Check sheet for the modelled part. Datum: model origin and axes. Units: mm. A direction names the side the tool comes from. Give positions to 0.01 mm unless a question says otherwise; leave off trailing zeros. Loops run counter-clockwise (first coordinate to the right, second up) from the corner with the lowest first, then second, coordinate; pieces in that order, holes last. Notation, with made-up numbers: (57.5, 81.5) - (110.5, 81.5) arc R30 ccw to (110.5, 110.5) - close; hole circle Ø3 at (-25.5, -28). An arc over 180 degrees is marked (long way). Use CSV: the item, a comma, the result in double quotes.
Autodesk Inventor part; units mm, degrees
ref_plane "ANBAU_XY" through (0, 0, -15.2) normal (0, -1, 0) x (1, 0, 0)
ref_plane "ANBAU_YZ" through (0, 0, -15.2) normal (1, 0, 0) x (0, 0, 1)
ref_plane "ANBAU_ZX" through (0, 0, -15.2) normal (0, 0, 1) x (0, -1, 0)
sketch "Sketch_1" plane through (0, 0, 0) normal (1, 0, 0) x (0, 1, 0)
  line L0 (22, 5.4) -> (-20.8, 5.4)
  arc A0 (-20.8, 5.4) -> (-21, 5.2) centre (-20.8, 5.2) ccw
  line L1 (-21, 5.2) -> (-21, 1.1788)
  arc A1 (-21, 1.1788) -> (-20.9463, 1.0424) centre (-20.8, 1.1788) ccw
  line L2 (-20.9463, 1.0424) -> (-20.419, 0.477)
  arc A2 (-20.419, 0.477) -> (-19.322, 0) centre (-19.322, 1.5) ccw
  line L3 (-19.322, 0) -> (21.2, 0)
  line L4 (21.2, 0) -> (21.2, -3.3)
  line L5 (21.2, -3.3) -> (21.6171, -3.3)
  line L6 (21.6171, -3.3) -> (22.1063, -2.2509)
  arc A3 (22.1063, -2.2509) -> (22.2, -1.8283) centre (21.2, -1.8283) ccw
  line L7 (22.2, -1.8283) -> (22.2, 5.2)
  arc A4 (22.2, 5.2) -> (22, 5.4) centre (22, 5.2) ccw
extrude "Extrusion1" add sketch "Sketch_1" along normal mid plane 8
sketch "Sketch_2" plane through (0, 0, 0) normal (1, 0, 0) x (0, 1, 0)
  line L0 (15, 4.2) -> (15, 5.4)
  line L1 (15, 5.4) -> (18.05, 5.4)
  line L2 (18.05, 5.4) -> (18.05, 4.2)
  line L3 (18.05, 4.2) -> (15, 4.2)
  line L4 (15, 4.2) -> (15, 5.4)
revolve "Revolution1" cut sketch "Sketch_2" angle 360 about axis through (0, 15, 4.2) along (0, 0, -1)
sketch "Sketch_3" plane through (0, 0, 0) normal (1, 0, 0) x (0, 1, 0)
  line L0 (-15, 4.2) -> (-15, 5.4)
  line L1 (-15, 5.4) -> (-11.95, 5.4)
  line L2 (-11.95, 5.4) -> (-11.95, 4.2)
  line L3 (-11.95, 4.2) -> (-15, 4.2)
  line L4 (-15, 4.2) -> (-15, 5.4)
revolve "Revolution2" cut sketch "Sketch_3" angle 360 about axis through (0, -15, 4.2) along (0, 0, -1)
sketch "Sketch_6" plane through (0, -21.6, 0) normal (0, 1, 0) x (1, 0, 0)
  arc A0 (-1.7301, -0.5774) -> (-2.6364, 0) centre (-2.6364, -1) ccw
  line L0 (-1.7301, -0.5774) -> (-1.2427, -1.6226)
  arc A1 (-1.2427, -1.6226) -> (-0.3364, -2.2) centre (-0.3364, -1.2) ccw
  line L1 (-0.3364, -2.2) -> (0.3364, -2.2)
  arc A2 (0.3364, -2.2) -> (1.2427, -1.6226) centre (0.3364, -1.2) ccw
  line L2 (1.2427, -1.6226) -> (1.7301, -0.5774)
  arc A3 (2.6364, 0) -> (1.7301, -0.5774) centre (2.6364, -1) ccw
  line L3 (2.6364, 0) -> (-2.6364, 0)
extrude "Extrusion2" cut sketch "Sketch_6" along normal blind 42.8
sketch "Sketch_4" plane through (0, 0, 0) normal (1, 0, 0) x (0, 1, 0)
  line L0 (15, -41.8) -> (15, 6.6)
  line L1 (15, 6.6) -> (16.6, 6.6)
  line L2 (16.6, 6.6) -> (17.471, 6.283)
  arc A0 (17.8, 5.8131) -> (17.471, 6.283) centre (17.3, 5.8131) ccw
  line L3 (17.8, 5.8131) -> (17.8, 4.2)
  line L4 (17.8, 4.2) -> (16.275, 4.2)
  line L5 (16.275, 4.2) -> (16.275, -34.575)
  line L6 (16.275, -34.575) -> (16.5, -34.8)
  line L7 (16.5, -34.8) -> (16.5, -41.4935)
  line L8 (16.5, -41.4935) -> (16.1935, -41.8)
  line L9 (16.1935, -41.8) -> (15, -41.8)
  line L10 (15, -41.8) -> (15, 6.6)
revolve "Revolution3" add sketch "Sketch_4" angle 360 about axis through (0, 15, -41.8) along (0, 0, -1)
thread "Thread1"
sketch "Sketch_5" plane through (0, 0, 0) normal (1, 0, 0) x (0, 1, 0)
  line L0 (-15, -41.8) -> (-15, 6.6)
  line L1 (-15, 6.6) -> (-13.4, 6.6)
  line L2 (-13.4, 6.6) -> (-12.529, 6.283)
  arc A0 (-12.2, 5.8131) -> (-12.529, 6.283) centre (-12.7, 5.8131) ccw
  line L3 (-12.2, 5.8131) -> (-12.2, 4.2)
  line L4 (-12.2, 4.2) -> (-13.725, 4.2)
  line L5 (-13.725, 4.2) -> (-13.725, -34.575)
  line L6 (-13.725, -34.575) -> (-13.5, -34.8)
  line L7 (-13.5, -34.8) -> (-13.5, -41.4935)
  line L8 (-13.5, -41.4935) -> (-13.8065, -41.8)
  line L9 (-13.8065, -41.8) -> (-15, -41.8)
  line L10 (-15, -41.8) -> (-15, 6.6)
revolve "Revolution4" add sketch "Sketch_5" angle 360 about axis through (0, -15, -41.8) along (0, 0, -1)
thread "Thread2"
sketch "Sketch_7" plane through (0, 15, 6.6) normal (0, 0, 1) x (0, 1, 0)
  line L0 (-1, -0.5774) -> (0, -1.1547)
  line L1 (0, -1.1547) -> (1, -0.5774)
  line L2 (1, -0.5774) -> (1, 0.5774)
  line L3 (1, 0.5774) -> (0, 1.1547)
  line L4 (0, 1.1547) -> (-1, 0.5774)
  line L5 (-1, 0.5774) -> (-1, -0.5774)
extrude "Extrusion3" cut sketch "Sketch_7" against normal blind 1.04
sketch "Sketch_8" plane through (0, -15, 6.6) normal (0, 0, 1) x (0, 1, 0)
  line L0 (-1, -0.5774) -> (0, -1.1547)
  line L1 (0, -1.1547) -> (1, -0.5774)
  line L2 (1, -0.5774) -> (1, 0.5774)
  line L3 (1, 0.5774) -> (0, 1.1547)
  line L4 (0, 1.1547) -> (-1, 0.5774)
  line L5 (-1, 0.5774) -> (-1, -0.5774)
extrude "Extrusion4" cut sketch "Sketch_8" against normal blind 1.04
sketch "Sketch_9" plane through (0, 0, 0) normal (0, 0, 1) x (1, 0, 0)
  line L0 (-5, -18.3964) -> (-5, -23.2)
  line L1 (-5, -23.2) -> (5, -23.2)
  line L2 (5, -23.2) -> (5, -18.3964)
  line L3 (5, -18.3964) -> (4, -18.3964)
  arc A0 (3.9732, -18.4964) -> (4, -18.3964) centre (3.8, -18.3964) ccw
  line L4 (3.9732, -18.4964) -> (1.8927, -22.1)
  arc A1 (1.7195, -22.2) -> (1.8927, -22.1) centre (1.7195, -22) ccw
  line L5 (1.7195, -22.2) -> (-1.7195, -22.2)
  arc A2 (-1.8927, -22.1) -> (-1.7195, -22.2) centre (-1.7195, -22) ccw
  line L6 (-1.8927, -22.1) -> (-3.9732, -18.4964)
  arc A3 (-4, -18.3964) -> (-3.9732, -18.4964) centre (-3.8, -18.3964) ccw
  line L7 (-4, -18.3964) -> (-5, -18.3964)
extrude "Extrusion5" cut sketch "Sketch_9" along normal blind 4
ref_plane "ANBAU_XY" through (0, 0, -15.2) normal (0, -1, 0) x (1, 0, 0)
ref_plane "ANBAU_YZ" through (0, 0, -15.2) normal (1, 0, 0) x (0, 0, 1)
ref_plane "ANBAU_ZX" through (0, 0, -15.2) normal (0, 0, 1) x (0, -1, 0)
ref_plane "ANBAU_2_XY" through (0, 0, -15.2) normal (1, 0, 0) x (0, 0, -1)
ref_plane "ANBAU_2_YZ" through (0, 0, -15.2) normal (0, 0, -1) x (0, 1, 0)
ref_plane "ANBAU_2_ZX" through (0, 0, -15.2) normal (0, 1, 0) x (1, 0, 0)
ref_plane "IP_ANBAU_XY" through (0, 0, 0) normal (0, 0, -1) x (1, 0, 0)
ref_plane "IP_ANBAU_YZ" through (0, 0, 0) normal (1, 0, 0) x (0, -1, 0)
ref_plane "IP_ANBAU_ZX" through (0, 0, 0) normal (0, -1, 0) x (0, 0, -1)
ref_plane "IP_ANBAU_2_XY" through (0, 0, -15.2) normal (1, 0, 0) x (0, 0, -1)
ref_plane "IP_ANBAU_2_YZ" through (0, 0, -15.2) normal (0, 0, -1) x (0, 1, 0)
ref_plane "IP_ANBAU_2_ZX" through (0, 0, -15.2) normal (0, 1, 0) x (1, 0, 0)
properties part number "8092760 MS4-MV-B---(46_high_m)"
1. Sectioned sample at B-B, the plane y = 19. Record the boundary of the cut face in (x, z).
Completed:
outline,"(-4, 0) - (-2.64, 0) arc R1 ccw to (-1.73, 0.58) - (-1.24, 1.62) arc R1 cw to (-0.34, 2.2) - (0.34, 2.2) arc R1 cw to (1.24, 1.62) - (1.73, 0.58) arc R1 ccw to (2.64, 0) - (4, 0) - (4, 5.4) - (-4, 5.4) - close"
2. Scan lines: line 1 along X through (y, z) = (-15, 5); line 2 along Z through (x, y) = (0.25, -1); line 3 along X through (y, z) = (-15, -8) (3 decimals). Record each from-to range of solid material in increasing order.
Completed:
line 1,"x = -4 to -3.05, -2.8 to 2.8, 3.05 to 4"
line 2,"z = 2.2 to 5.4"
line 3,"x = -1.275 to 1.275"
3. Set-up check for faces 4 (the face through (0.07, 13.5, -38.19)), 5 (the face through (1, -16, 6.6)), 6 (the face through (-0.87, -15.49, 6.09)): record each of +Z, -Z, +X, -X, +Y, -Y from which the full face is reachable in a straight line by a thin tool's end or side.
Completed:
face 4,"-Z"
face 5,"+Z, +X, -X, +Y, -Y"
face 6,"+Z"
4. Release check for a two-part mould opening along X. For faces 1 (the face through (1, 14, 6.6)), 2 (the face through (0.1, -17.8, 5)), 3 (the face through (-3.24, -19.77, 1.97)) record: released by +X, released by -X, zero draft, split by the parting line, or undercut.
Completed:
face 1,"zero draft"
face 2,"undercut"
face 3,"released by -X"
5. Go/stop test with flat-tipped pins: pin 1 Ø2.5 at (x, y) = (0.5, 4.5) entering from +Z; pin 2 Ø1.6 at (x, y) = (0, -15) entering from +Z; pin 3 Ø1.6 at (x, z) = (1.5, 0.5) entering from -Y; pin 4 Ø0.5 at (x, z) = (0, 6) entering from -Y. Record where each tip stops, or that it passes through.
Completed:
pin 1,"stops at z = 5.4"
pin 2,"stops at z = 5.56"
pin 3,"stops at y = -21"
pin 4,"stops at y = -17.8"
6. Sectioned sample at A-A, the plane z = -24.5. Record the boundary of the cut face in (x, y) (3 decimals), and give its area (3 significant figures).
Completed:
outline,"circle Ø2.55 at (0, -15); circle Ø2.55 at (0, 15)"
area,"10.2 mm²"
